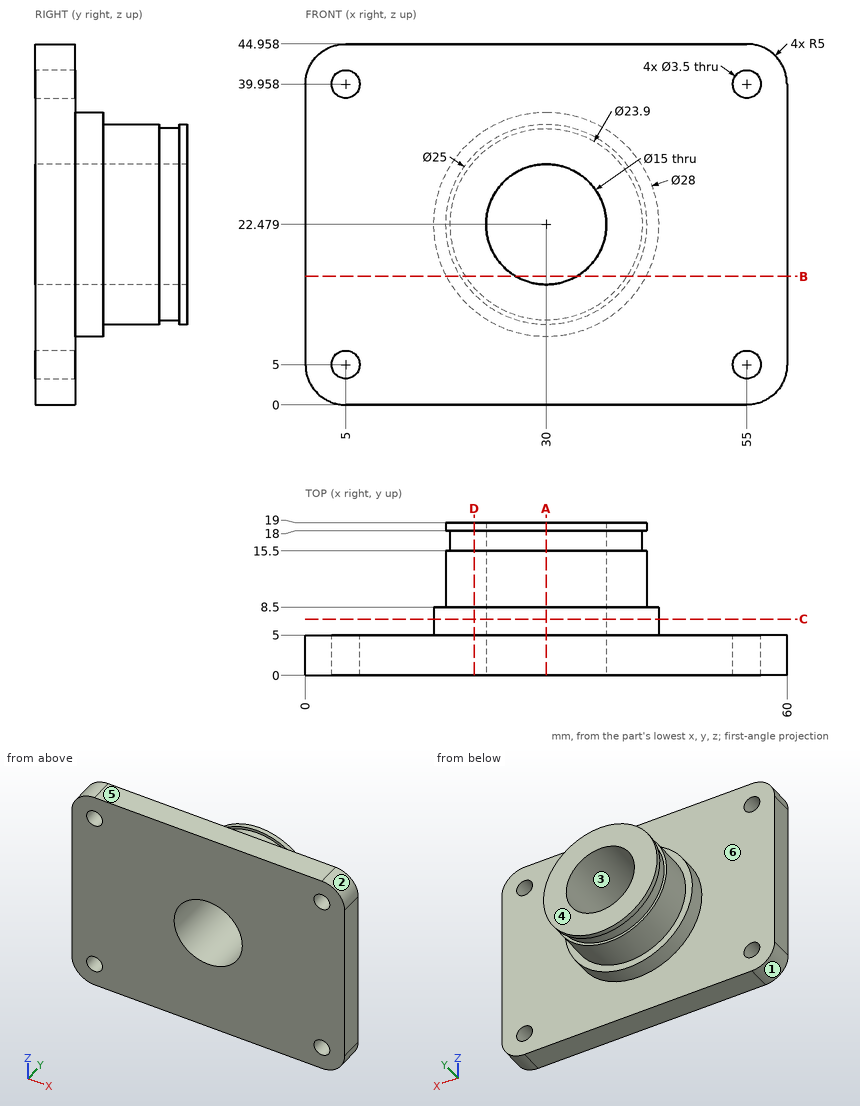
Study the drawing (mm; zero at the part's minimum x, y, z) and answer. A direction names the side the tool comes from. Give positions to 0.01 mm unless a question says otherwise; leave off trailing zeros. Write each loop counter-clockwise with the first axis right and the second up, starting at its lowest first coordinate (ties: lowest second). Pieces come first, ordered by that corner, then holes.
Item 1: Section D-D, the plane x = 21 is taken. Write down the section's boundary in (y, z).
Item 2: Section A-A, the plane x = 30 is taken. Write down the section's boundary in (y, z).
Item 3: Which of the six approach directions +Z, -Z, +X, -X, +Y, -Y give full straight-line access (tool end or side, diameter ignored) to the marked faces 5 and 6?
Item 4: Section B-B, the plane z = 16 is taken. Write down the section's boundary in (x, y).
Item 5: Find the intervals of material crossed by line 1 along X through (y, z) = (3.25, 5); line 2 along Z through (x, y) = (30, 12.5); line 3 along Y through (x, z) = (18, 14.5), in increasing order.
Item 6: Determine the mould class of the marked faces 1, 2, 3 and 4 for opening direction Z: released by +Z, released by -Z, zero draft, split by the parting line, or undercut.
Item 7: Flat-ended cylindrical pins translate along their axes: P1, Ø4, axis at y = 14.5, z = 26, coming from the -X side; P2, Ø6, axis at x = 9, z = 17, coming from the +Y side; P3, Ø2, axis at x = 5, z = 5, coming from the +Y side; P4, Ø8, axis at x = 39, y = 11.5, coming from the +Z side. Find the tip coordinate at first contact, or state that the pin passes through.
Item 8: Section C-C, the plane y = 7 is taken. Write down the section's boundary in (x, z), plus the area to 3 significant figures.
Completed:
1. outline: (0, 0) - (5, 0) - (5, 11.76) - (8.5, 11.76) - (8.5, 13.8) - (15.5, 13.8) - (15.5, 14.62) - (18, 14.62) - (18, 13.8) - (19, 13.8) - (19, 31.15) - (18, 31.15) - (18, 30.34) - (15.5, 30.34) - (15.5, 31.15) - (8.5, 31.15) - (8.5, 33.2) - (5, 33.2) - (5, 44.96) - (0, 44.96) - close
2. outline: (0, 0) - (5, 0) - (5, 8.48) - (8.5, 8.48) - (8.5, 9.98) - (15.5, 9.98) - (15.5, 10.53) - (18, 10.53) - (18, 9.98) - (19, 9.98) - (19, 14.98) - (0, 14.98) - close; (0, 29.98) - (19, 29.98) - (19, 34.98) - (18, 34.98) - (18, 34.43) - (15.5, 34.43) - (15.5, 34.98) - (8.5, 34.98) - (8.5, 36.48) - (5, 36.48) - (5, 44.96) - (0, 44.96) - close
3. face 5: +Z, +X, -X, +Y, -Y
3. face 6: +Y
4. outline: (0, 0) - (26.22, 0) - (26.22, 19) - (19.31, 19) - (19.31, 18) - (19.96, 18) - (19.96, 15.5) - (19.31, 15.5) - (19.31, 8.5) - (17.59, 8.5) - (17.59, 5) - (0, 5) - close; (33.78, 0) - (60, 0) - (60, 5) - (42.41, 5) - (42.41, 8.5) - (40.69, 8.5) - (40.69, 15.5) - (40.04, 15.5) - (40.04, 18) - (40.69, 18) - (40.69, 19) - (33.78, 19) - close
5. line 1: x = 0 to 3.25, 6.75 to 53.25, 56.75 to 60
5. line 2: z = 9.98 to 14.98, 29.98 to 34.98
5. line 3: y = 0 to 5
6. face 1: released by -Z
6. face 2: released by +Z
6. face 3: undercut
6. face 4: zero draft
7. P1: stops at x = 17.59
7. P2: stops at y = 5
7. P3: passes through
7. P4: stops at z = 34.95
8. outline: circle Ø28 at (30, 22.48); hole circle Ø15 at (30, 22.48)
8. area: 439 mm2
